from build123d import *

# Parameters (mm, degrees)
F0_R     = 2.5
F0_R_2   = 22.5
F1_DEPTH = 6


with BuildPart() as f1:
    # F0 (on Front) → F1 (new body)
    with BuildSketch(Plane.XZ):
        with BuildLine():
            ThreePointArc((-10.045547, 56.971129), (-37.185263, -44.315671), (57.85, 0))
            ThreePointArc((57.85, 0), (37.185263, 44.315671), (-10.045547, 56.971129))
        make_face()
        with Locations((-21.5, -37.239092)):
            Circle(F0_R, mode=Mode.SUBTRACT)
        with BuildLine():
            ThreePointArc((-23.382686, 13.5), (-24.368717, 11.626075), (-25.204864, 9.680642))
            ThreePointArc((-25.204864, 9.680642), (-27, 0), (-25.204864, -9.680642))
            ThreePointArc((-25.204864, -9.680642), (-24.368717, -11.626075), (-23.382686, -13.5))
            ThreePointArc((-23.382686, -13.5), (-23.262708, -13.705708), (-23.14092, -13.91035))
            ThreePointArc((-23.14092, -13.91035), (-22.49477, -17.311118), (-24.212337, -20.316563))
            Line((-24.212337, -20.316563), (-34.258549, -28.746336))
            ThreePointArc((-34.258549, -28.746336), (-38.184741, -29.865123), (-41.636097, -27.684571))
            ThreePointArc((-41.636097, -27.684571), (-42.489891, -26.35544), (-43.30127, -25))
            ThreePointArc((-43.30127, -25), (-44.625232, -22.551911), (-45.810926, -20.033948))
            ThreePointArc((-45.810926, -20.033948), (-50, 0), (-45.810926, 20.033948))
            ThreePointArc((-45.810926, 20.033948), (-44.625232, 22.551911), (-43.30127, 25))
            ThreePointArc((-43.30127, 25), (-42.489891, 26.35544), (-41.636097, 27.684571))
            ThreePointArc((-41.636097, 27.684571), (-38.184741, 29.865123), (-34.258549, 28.746336))
            Line((-34.258549, 28.746336), (-24.212337, 20.316563))
            ThreePointArc((-24.212337, 20.316563), (-22.49477, 17.311118), (-23.14092, 13.91035))
            ThreePointArc((-23.14092, 13.91035), (-23.262708, 13.705708), (-23.382686, 13.5))
        make_face(mode=Mode.SUBTRACT)
        Circle(F0_R_2, mode=Mode.SUBTRACT)
        with BuildLine():
            ThreePointArc((4.21875, -26.668374), (13.5, -23.382686), (20.986114, -16.987731))
            ThreePointArc((20.986114, -16.987731), (22.252835, -15.29089), (23.382686, -13.5))
            ThreePointArc((23.382686, -13.5), (23.500845, -13.293242), (23.617176, -13.085449))
            ThreePointArc((23.617176, -13.085449), (26.239253, -10.825483), (29.700828, -10.810217))
            Line((29.700828, -10.810217), (42.024332, -15.295606))
            ThreePointArc((42.024332, -15.295606), (44.956326, -18.136394), (44.79359, -22.215632))
            ThreePointArc((44.79359, -22.215632), (44.069426, -23.619605), (43.30127, -25))
            ThreePointArc((43.30127, -25), (41.843144, -27.370629), (40.255371, -29.656452))
            ThreePointArc((40.255371, -29.656452), (25, -43.30127), (5.555556, -49.690399))
            ThreePointArc((5.555556, -49.690399), (2.782088, -49.92254), (0, -50))
            ThreePointArc((0, -50), (-1.579535, -49.975044), (-3.157493, -49.900203))
            ThreePointArc((-3.157493, -49.900203), (-6.771585, -48.001517), (-7.765783, -44.041942))
            Line((-7.765783, -44.041942), (-5.488491, -31.12678))
            ThreePointArc((-5.488491, -31.12678), (-3.744483, -28.136601), (-0.476257, -26.995799))
            ThreePointArc((-0.476257, -26.995799), (-0.238138, -26.99895), (0, -27))
            ThreePointArc((0, -27), (2.115882, -26.916966), (4.21875, -26.668374))
        make_face(mode=Mode.SUBTRACT)
        with BuildLine():
            ThreePointArc((40.5, 0), (43, 2.5), (45.5, 0))
            ThreePointArc((45.5, 0), (43, -2.5), (40.5, 0))
        make_face(mode=Mode.SUBTRACT)
        with Locations((-21.5, 37.239092)):
            Circle(F0_R, mode=Mode.SUBTRACT)
        with BuildLine():
            ThreePointArc((20.986114, 16.987731), (13.5, 23.382686), (4.21875, 26.668374))
            ThreePointArc((4.21875, 26.668374), (1.878394, 26.934581), (-0.476257, 26.995799))
            ThreePointArc((-0.476257, 26.995799), (-3.744483, 28.136601), (-5.488491, 31.12678))
            Line((-5.488491, 31.12678), (-7.765783, 44.041942))
            ThreePointArc((-7.765783, 44.041942), (-6.771585, 48.001517), (-3.157493, 49.900203))
            ThreePointArc((-3.157493, 49.900203), (1.203611, 49.985511), (5.555556, 49.690399))
            ThreePointArc((5.555556, 49.690399), (25, 43.30127), (40.255371, 29.656452))
            ThreePointArc((40.255371, 29.656452), (42.686917, 26.035114), (44.79359, 22.215632))
            ThreePointArc((44.79359, 22.215632), (44.956326, 18.136394), (42.024332, 15.295606))
            Line((42.024332, 15.295606), (29.700828, 10.810217))
            ThreePointArc((29.700828, 10.810217), (26.239253, 10.825483), (23.617176, 13.085449))
            ThreePointArc((23.617176, 13.085449), (22.386834, 15.094028), (20.986114, 16.987731))
        make_face(mode=Mode.SUBTRACT)
    extrude(amount=F1_DEPTH)


solid = f1.part
Check sheet for the modelled part. Datum: model origin and axes. Units: mm. A direction names the side the tool comes from. Round coordinates to 2 decimals unless told otherwise and drop trailing zeros. Loops run counter-clockwise (first coordinate to the right, second up) from the corner with the lowest first, then second, coordinate; pieces in that order, holes last.
1. Sectioned sample at A-A on x = 12. Record the boundary of the cut face in (y, z), and give its area (3 significant figures).
2. Sectioned sample at B-B on z = -8. Record the boundary of the cut face in (x, y).
3. Gauge pin test, flat ends, axial feed: pin 1 Ø1.5 at (y, z) = (-3.5, -23.5) entering from -X; pin 2 Ø1 at (x, y) = (5.5, -5) entering from -Z; pin 3 Ø2 at (x, y) = (-44.5, -4) entering from +Z. Record the tip position at first contact, or that the pin passes through.
4. Mould release check, pull along Z, two halves, no side actions. Record for faces 1 (the flat face through (-1, 0, -25)), 2 (the cylindrical face through (44.08, -2.96, -23.6)): released by +Z, released by -Z, zero draft, split by the parting line, or undercut.
5. Scan lines: probe 1 along Z at (x, y) = (1, -1.35); probe 2 along Z at (x, y) = (40, -5); probe 3 along X at (y, z) = (-4.1, -3.5). Record each from-to range of solid material in increasing order.
6. Sectioned sample at C-C on y = -4.05. Give the number of separate pieces and of enclosed holes in the cut face, and give its area (3 significant figures).
7. Set-up check for faces 3 (the flat face through (-6.643, -2.958, -37.675)), 4 (the flat face through (-1, -6, -25)): record each of +Z, -Z, +X, -X, +Y, -Y from which the full face is reachable in a straight line by a thin tool's end or side.
Recorded:
1. outline: (-6, -56.59) - (0, -56.59) - (0, -48.54) - (-6, -48.54) - close; (-6, -24.19) - (0, -24.19) - (0, -19.03) - (-6, -19.03) - close; (-6, 19.03) - (0, 19.03) - (0, 24.19) - (-6, 24.19) - close; (-6, 48.54) - (0, 48.54) - (0, 56.59) - (-6, 56.59) - close
1. area: 158 mm2
2. outline: (-57.29, -6) - (-49.36, -6) - (-49.36, 0) - (-57.29, 0) - close; (-25.79, -6) - (-21.03, -6) - (-21.03, 0) - (-25.79, 0) - close; (21.03, -6) - (57.29, -6) - (57.29, 0) - (21.03, 0) - close
3. pin 1: stops at x = -53.19
3. pin 2: stops at z = -57.63
3. pin 3: stops at z = 38.14
4. face 1: zero draft
4. face 2: undercut
5. probe 1: z = -57.84 to -49.99, -26.98 to -22.48, 22.48 to 26.98, 49.99 to 57.84
5. probe 2: z = -41.79 to -30, -14.56 to 14.56, 30 to 41.79
5. probe 3: x = -57.74 to -49.88, -26.77 to -22.23, 22.23 to 57.74
6. separate pieces: 1
6. enclosed holes: 7
6. area: 5,220 mm2
7. face 3: +Y, -Y
7. face 4: +Z, -Z, +X, -X, -Y
